Geometry check sheet. Reference: the model listing, model coordinates, mm. A direction names the side the tool comes from. Coordinates: 2 decimals unless noted, no trailing zeros. Write each loop counter-clockwise with the first axis right and the second up, starting at its lowest first coordinate (ties: lowest second). Pieces come first, ordered by that corner, then holes.
from build123d import *

# Parameters (mm, degrees)
BOSS_EXTRUDE2_DEPTH = 30
FILLET1_R           = 10
SKETCH3_R           = 10
CUT_EXTRUDE1_DEPTH  = 187.815416923


with BuildPart() as part:
    # Sketch2 → Boss-Extrude2 (new body)
    with BuildSketch(Plane.XY):
        Polygon((0, 0), (0, 10), (-40, 10), (-40, 0), (-140, 0), (-140, 10), (-180, 10), (-180, -30), (-140, -30), (-140, -20), (-40, -20), (-40, -30), (0, -30), align=None)
    extrude(amount=BOSS_EXTRUDE2_DEPTH)

    # Fillet1
    fillet1_edges = [part.edges().sort_by_distance(p)[0] for p in [
        (-40, -20, 15),
        (-140, -20, 15),
        (-40, 0, 15),
        (-140, 0, 15),
    ]]
    fillet(fillet1_edges, radius=FILLET1_R - 0.0001)  # a hair under: the kernel refuses the full size

    # Sketch3 → Cut-Extrude1 (cut, through all)
    with BuildSketch(Plane(origin=(0, 10, 0), x_dir=(1, 0, 0), z_dir=(0, 1, 0))):
        with Locations(Location((-20, -15, 0), (0, 0, 180))):
            Circle(SKETCH3_R)
        with Locations((-200, -15)):
            Circle(SKETCH3_R)
    extrude(amount=-CUT_EXTRUDE1_DEPTH, mode=Mode.SUBTRACT)


solid = part.part
1. Sectioned sample at A-A, the plane x = -20. Record the boundary of the cut face in (y, z).
Computed values:
outline: (-30, 0) - (10, 0) - (10, 5) - (-30, 5) - close; (-30, 25) - (10, 25) - (10, 30) - (-30, 30) - close
2. Sectioned sample at B-B, the plane y = -26. Record the boundary of the cut face in (x, z).
Computed values:
outline: (-180, 0) - (-139.17, 0) - (-139.17, 30) - (-180, 30) - close; (-40.83, 0) - (0, 0) - (0, 30) - (-40.83, 30) - close; hole circle Ø20 at (-20, 15)
3. Access from +Z, -Z, +X, -X, +Y, -Y to the whole of each face (thin tool, end or side, straight path). Record for faces 4 (the flat face through (-160, 10, 15)), 5 (the flat face through (-89, 0, 15)), 6 (the cylindrical face through (-137.15, -23.01, 15.21)).
Computed values:
face 4: +Z, -Z, +X, -X, +Y
face 5: +Z, -Z, +Y
face 6: +Z, -Z, -Y
4. Thickness scan on line 1 along Z through (x, y) = (-20, -5.5); line 2 along Z through (x, y) = (-18, 0.5); line 3 along X through (y, z) = (-25, 17.75). Record the ranges inside material, lowest first.
Computed values:
line 1: z = 0 to 5, 25 to 30
line 2: z = 0 to 5.2, 24.8 to 30
line 3: x = -180 to -138.66, -41.34 to -29.61, -10.39 to 0
5. Gauge pin test, flat ends, axial feed: pin 1 Ø3 at (x, z) = (-111.5, 12.5) entering from -Y; pin 2 Ø2 at (x, z) = (-137, 17.5) entering from +Y. Record the tip position at first contact, or that the pin passes through.
Computed values:
pin 1: stops at y = -20
pin 2: stops at y = 4
6. Draft check along X on faces 1 (the flat face through (-91, -20, 15)), 2 (the flat face through (-180, -10, 15)), 3 (the flat face through (-91, -10, 30)). Enter one of: released by +X, released by -X, zero draft, split by the parting line, or undercut.
Computed values:
face 1: undercut
face 2: released by -X
face 3: zero draft
7. Sectioned sample at D-D, the plane y = -3. Record the boundary of the cut face in (x, z), and give its area (3 significant figures).
Computed values:
outline: (-180, 0) - (0, 0) - (0, 30) - (-180, 30) - close; hole circle Ø20 at (-20, 15)
area: 5,090 mm2
